Source: CAD feature listing. Evaluate the final solid. Frame: model axes, mm. Round coordinates to 2 decimals unless told otherwise and drop trailing zeros. Loops run counter-clockwise (first coordinate to the right, second up) from the corner with the lowest first, then second, coordinate; pieces in that order, holes last.
(1) Material intervals for probe 1 along Y at (x, z) = (-325.25, 221.5); probe 2 along Y at (x, z) = (-330, 227.5); probe 3 along Y at (x, z) = (-330, 272), sorted ascending.
(2) First-contact query: pin 1 Ø1.5 at (x, y) = (-327, 33) entering from -Z; pin 2 Ø0.6 at (x, y) = (-329, 19.5) entering from +Z; pin 3 Ø2 at (y, z) = (28, 228.5) entering from -X; pin 4 Ø3 at (x, y) = (-328, 39.5) entering from +Z. Flat tips, straight axial feed; report the tip coordinate or a pass-through.
(3) Section D-D, the plane y = 26. Return the cut outline in (x, z), plus the area to 3 significant figures.
(4) Section C-C, the plane y = 35. Return the cut outline in (x, z).
(5) Section A-A, the plane z = 229.5. Return the cut outline in (x, y), plus the area to 3 significant figures.
(6) Mould query, pull axis Y, two halves, no side actions, for faces 1 (the flat face through (-328, 25, 209.836)), 2 (the flat face through (-328, 32, 215.836)). Classes: pulls with the +Y half, pulls with the -Y half, needs draft (parallel to the pull), parting line crosses it, or undercut.
(7) Section B-B, the plane z = 258.5. Return the cut outline in (x, y), plus the area to 3 significant figures.
Autodesk Inventor part; units mm, degrees
ref_plane "РабПлоскость1" through (-327.803629, 8.784154, 215.836479) normal (0, 0, 1) x (1, 0, 0)
ref_plane "РабПлоскость2" through (-327.498735, 8.403036, 292.836479) normal (0, 0, -1) x (-0.999864, -0.0164918, 0)
ref_plane "РабПлоскость3" through (-672.954973, 50.067364, -86.377936) normal (-0.0164918, 0.999864, 0) x (0, 0, 1)
ref_plane "РабПлоскость1" through (-327.803629, 8.784154, 215.836479) normal (0, 0, 1) x (1, 0, 0)
sketch "Эскиз1" plane through (-327.803629, 8.784154, 215.836479) normal (0, 0, 1) x (1, 0, 0)
  line L0 (3.114831, 11.166777) -> (2.944416, 21.498705)
  line L1 (2.944416, 21.498705) -> (-3.054768, 21.399754)
  line L2 (-3.054768, 21.399754) -> (-2.884353, 11.067826)
  line L3 (-2.884353, 11.067826) -> (3.114831, 11.166777)
  line L4 (-3.393221, 41.919489) -> (-3.225183, 31.731682)
  line L5 (2.774001, 31.830633) -> (2.605963, 42.01844)
  line L6 (-3.225183, 31.731682) -> (2.774001, 31.830633)
  line L7 (2.605963, 42.01844) -> (-3.393221, 41.919489)
  line L8 (2.774001, 31.830633) -> (2.605963, 42.01844) construction
  line L9 (-3.393221, 41.919489) -> (-3.225183, 31.731682) construction
  line L10 (3.114831, 11.166777) -> (2.944416, 21.498705) construction
  line L11 (-3.054768, 21.399754) -> (-2.884353, 11.067826) construction
  line L12 (6.149374, 48.077701) -> (19.433282, 48.296806) construction
  line L13 (2.605963, 42.01844) -> (6.248325, 42.078517) construction
  point P0 (327.803629, -8.784154)
  dimension "d16" = 6
extrude "Выдавливание1" add sketch "Эскиз1" against normal blind 6
ref_plane "РабПлоскость2" through (-327.498735, 8.403036, 292.836479) normal (0, 0, -1) x (-0.999864, -0.0164918, 0)
sketch "Эскиз2" plane through (-327.498735, 8.403036, 292.836479) normal (0, 0, -1) x (-0.999864, -0.0164918, 0)
  line L0 (-3, 21.833317) -> (3, 21.833317)
  line L1 (3, 21.833317) -> (3, 11.499984)
  line L2 (3, 11.5) -> (-3, 11.5)
  line L3 (-3, 11.499984) -> (-3, 21.833317)
  line L4 (3, 32.16665) -> (-3, 32.16665)
  line L5 (-3, 32.16665) -> (-3, 42.355843)
  line L6 (-3, 42.5) -> (3, 42.5)
  line L7 (3, 42.355843) -> (3, 32.16665)
  line L8 (-3, 11.499984) -> (-3, 21.833317) construction
  line L9 (3, 21.833317) -> (3, 11.499984) construction
  line L10 (-3, 32.16665) -> (-3, 42.355843) construction
  line L11 (3, 42.355843) -> (3, 32.16665) construction
  point P0 (-327.315615, -13.802923)
sketch "Эскиз2 outline for Выдавливание2" plane through (-327.498735, 8.403036, 292.836479) normal (0, 0, -1) x (-0.999864, -0.0164918, 0)
  line L0 (3, 32.16665) -> (3, 42.355843)
  line L1 (-3, 32.16665) -> (3, 32.16665)
  line L2 (-3, 42.355843) -> (-3, 32.16665)
  line L3 (3, 42.355843) -> (-3, 42.355843)
  line L4 (-3, 21.833317) -> (-3, 11.499984)
  line L5 (3, 21.833317) -> (-3, 21.833317)
  line L6 (3, 11.499984) -> (3, 21.833317)
  line L7 (-3, 11.499984) -> (3, 11.499984)
extrude "Выдавливание2" add sketch "Эскиз2 outline for Выдавливание2" against normal blind 6
sketch "Эскиз3" plane through (-327.498735, 8.403036, 292.836479) normal (0, 0, -1) x (-0.999864, -0.0164918, 0)
  circle A0 centre (0, -7.644157) radius 18
  line L0 (6.642857, 42.355843) -> (3, 42.355843)
  line L1 (-3, 32.166667) -> (-3, 21.833333)
  line L2 (-3, 21.833333) -> (3, 21.833333)
  line L3 (3, 21.833333) -> (3, 32.166667)
  line L4 (3, 32.166667) -> (-3, 32.166667)
  line L5 (-3, 42.355843) -> (3, 42.355843)
  line L6 (3, 42.355843) -> (3, 10.355843)
  line L7 (3, 10.355843) -> (-3, 10.355843)
  line L8 (-3, 10.355843) -> (-3, 42.355843)
  point P0 (-327.315615, -13.802923)
  point P1 (-3, 21.833333)
  point P2 (3, 21.833333)
  point P3 (3, 42.355843)
extrude "Выдавливание3" add sketch "Эскиз3" along normal up to surface (77 mm away) contours L7 L8 L2 L6 | L2 L1 L4 L3 | L4 L8 L5 L6
sketch "Эскиз4" plane through (-331.19685, 50.703643, 209.836479) normal (-0.999864, -0.0164918, 0) x (0, 0, 1)
  line L0 (0, -14) -> (6, -14) construction
  line L1 (0, -17) -> (6, -17) construction
  line L2 (6, -17) -> (6, -14)
  line L3 (6, -14) -> (12.35, -14)
  line L4 (12.35, -14) -> (12.35, -12.75)
  line L5 (12.35, -12.75) -> (14.65, -12.75)
  line L6 (14.65, -12.75) -> (14.65, -14)
  line L7 (14.65, -14) -> (21, -14)
  line L8 (21, -14) -> (21, -17)
  line L9 (21, -17) -> (14.65, -17)
  line L10 (14.65, -17) -> (14.65, -18.25)
  line L11 (14.65, -18.25) -> (12.35, -18.25)
  line L12 (12.35, -18.25) -> (12.35, -17)
  line L13 (12.35, -17) -> (6, -17)
  line L14 (0, -20.522506) -> (0, -30.855843) construction
  line L15 (89, -10.189193) -> (89, 0) construction
  line L16 (0, -30.855843) -> (89, 0) construction
  line L17 (44.5, 0) -> (44.5, -30.855843) construction
  line L18 (89, -14) -> (83, -14) construction
  line L19 (89, -17) -> (83, -17) construction
  line L20 (83, -17) -> (83, -14)
  line L21 (83, -14) -> (76.65, -14)
  line L22 (76.65, -14) -> (76.65, -12.75)
  line L23 (76.65, -12.75) -> (74.35, -12.75)
  line L24 (74.35, -12.75) -> (74.35, -14)
  line L25 (74.35, -14) -> (68, -14)
  line L26 (68, -14) -> (68, -17)
  line L27 (68, -17) -> (74.35, -17)
  line L28 (74.35, -17) -> (74.35, -18.25)
  line L29 (74.35, -18.25) -> (76.65, -18.25)
  line L30 (76.65, -18.25) -> (76.65, -17)
  line L31 (76.65, -17) -> (83, -17)
  point P0 (-209.836479, -56.158766)
  point P1 (44.5, -15.427922)
  dimension "d9" = 2.3
  dimension "d10" = 5.5
  dimension "d11" = 15
extrude "Выдавливание4" cut sketch "Эскиз4" against normal blind 6
ref_plane "РабПлоскость3" through (-672.954973, 50.067364, -86.377936) normal (-0.0164918, 0.999864, 0) x (0, 0, 1)
sketch "Эскиз5" plane through (-331.19685, 50.703643, 292.636479) normal (-0.0164918, 0.999864, 0) x (0.999864, 0.0164918, 0)
  line L0 (6, 51.133333) -> (6, 25.466667)
  line L1 (0, 51.133333) -> (6, 51.133333)
  line L2 (0, 25.466667) -> (0, 51.133333)
  line L3 (6, 25.466667) -> (0, 25.466667)
  point P0 (330.315615, 292.636479)
extrude "Выдавливание5" add sketch "Эскиз5" along normal up to surface (5 mm away)
equation "\"d1\" = d0"
equation "\"d3\" = d0"
equation "\"d7\" = d0"
equation "\"d12\" = d3"
equation "\"d0\" = d16"
properties part number "motor1"
Output values:
1. probe 1: y = 18.8 to 33.8, 36.8 to 50.8
1. probe 2: y = 18.72 to 33.72, 36.72 to 50.72
1. probe 3: y = 18.72 to 50.72
2. pin 1: stops at z = 215.84
2. pin 2: stops at z = 292.84
2. pin 3: stops at x = -330.84
2. pin 4: stops at z = 298.84
3. outline: (-330.79, 209.84) - (-324.79, 209.84) - (-324.79, 298.84) - (-330.79, 298.84) - close
3. area: 534 mm2
4. outline: (-330.94, 230.84) - (-324.94, 230.84) - (-324.94, 277.84) - (-330.94, 277.84) - close
5. outline: (-331.2, 50.7) - (-330.97, 36.71) - (-324.97, 36.8) - (-325.2, 50.8) - close; (-330.92, 33.71) - (-330.67, 18.71) - (-324.67, 18.81) - (-324.92, 33.8) - close
5. area: 174 mm2
6. face 1: needs draft
6. face 2: undercut
7. outline: (-331.28, 55.7) - (-330.67, 18.71) - (-324.67, 18.81) - (-325.28, 55.8) - close
7. area: 222 mm2
